```python
from build123d import *

# Parameters (mm, degrees)
F0_W     = 106.6328883171
F0_H     = 89.0891589573
F1_DEPTH = 11.1428909004
F3_DEPTH = 37.5499762595
F6_DEPTH = 6.3658682629


with BuildPart() as f1:
    # F0 (on Top) → F1 (new body)
    with BuildSketch(Plane.XY):
        Rectangle(F0_W, F0_H)
    extrude(amount=F1_DEPTH)

    # F2 (on face) → F3 (join)
    with BuildSketch(Plane(origin=(-53.3164441586, 0, 0), x_dir=(0, -1, 0), z_dir=(-1, 0, 0))):
        Polygon((5.0119608641, 11.1428909004), (44.5445794787, 11.1428909004), (44.5445794787, 33.9670588993), align=None)
    extrude(amount=-F3_DEPTH)

    # F4: F1 across plane


with BuildPart() as f1_1:
    add(f1.part)
    add(f1.part.mirror(Plane.YZ))

    # F5 (on face) → F6 (join)
    with BuildSketch(Plane.XY.offset(11.1428909004)):
        Polygon((-15.7664678991, -5.0119608641), (-15.7664678991, -44.5445794787), (15.7664678991, -44.5445794787), (15.7664678991, -5.0119608641), (15.7664678991, 44.5445794787), (-15.7664678991, 44.5445794787), align=None)
    extrude(amount=F6_DEPTH)


solid = f1_1.part
```
CAD build for the part. Positions are in the model's coordinates, mm. A direction names the side the tool comes from. Round coordinates to 2 decimals unless told otherwise and drop trailing zeros. Order: outer loops, then holes, each group sorted by start corner. A loop starts at its lowest first (then second) coordinate and runs counter-clockwise, first axis right, second up.
Q1. Which spindle directions (+Z, -Z, +X, -X, +Y, -Y) get a long thin tool onto all of the face, cutting with end or side? Do faces 1 (the flat face through (-1, -44.545, 17)), 2 (the flat face through (34, 20, 11.143)), 3 (the flat face through (-15.766, -36, 22)), 4 (the flat face through (-35, 20, 11.143)). Say none if no direction does.
Q2. Slice it at A-A (z = 22). Write the cut outline in (x, y).
Q3. Slice it at B-B (y = 0.5). Write the cut outline in (x, z), and give its area (3 significant figures).
Q4. Wall check: L1, parallel to X at y = -28.5, z = 20; L2, parallel to Z at x = 20.5, y = 0.5; L3, parallel to Z at x = -9, y = -28. Give the ranges that are in metal, low to high.
Q5. Two-plate mould, pull along X, no slides. Class faces 5 (the flat face through (34.8, -25.05, 22.71)), 6 (the flat face through (15.766, -36, 22)), 7 (the flat face through (15.766, 14, 14)): pulls with the +X half, pulls with the -X half, needs draft (parallel to the pull), parting line crosses it, or undercut.
Q6. Drop flat-ended pins along their axis: pin 1 (10 mm diameter, centred on x = 37, y = 33.5, fed in from +Z); pin 2 (7 mm diameter, centred on y = 26, z = 15.5, fed in from +X); pin 3 (5 mm diameter, centred on y = 27, z = 14, fed in from -X). Give the stop position or say it passes through.
Q7. Slice it at C-C (x = 38.5). Write the cut outline in (y, z).
Q8. Slice it at D-D (z = 12.5). Write the cut outline in (x, y).
Results below:
1. face 1: +Z, -Z, +X, -X, -Y
1. face 2: +Z, +X, +Y
1. face 3: +Z, +Y, -Y
1. face 4: +Z, -X, +Y
2. outline: (-53.32, -44.54) - (-15.77, -44.54) - (-15.77, -23.82) - (-53.32, -23.82) - close; (15.77, -44.54) - (53.32, -44.54) - (53.32, -23.82) - (15.77, -23.82) - close
3. outline: (-53.32, 0) - (53.32, 0) - (53.32, 11.14) - (15.77, 11.14) - (15.77, 17.51) - (-15.77, 17.51) - (-15.77, 11.14) - (-53.32, 11.14) - close
3. area: 1,390 mm2
4. L1: x = -53.32 to -15.77, 15.77 to 53.32
4. L2: z = 0 to 11.14
4. L3: z = 0 to 17.51
5. face 5: needs draft
5. face 6: undercut
5. face 7: pulls with the +X half
6. pin 1: stops at z = 11.14
6. pin 2: stops at x = 15.77
6. pin 3: stops at x = -15.77
7. outline: (-44.54, 0) - (44.54, 0) - (44.54, 11.14) - (-5.01, 11.14) - (-44.54, 33.97) - close
8. outline: (-53.32, -44.54) - (53.32, -44.54) - (53.32, -7.36) - (15.77, -7.36) - (15.77, 44.54) - (-15.77, 44.54) - (-15.77, -7.36) - (-53.32, -7.36) - close
